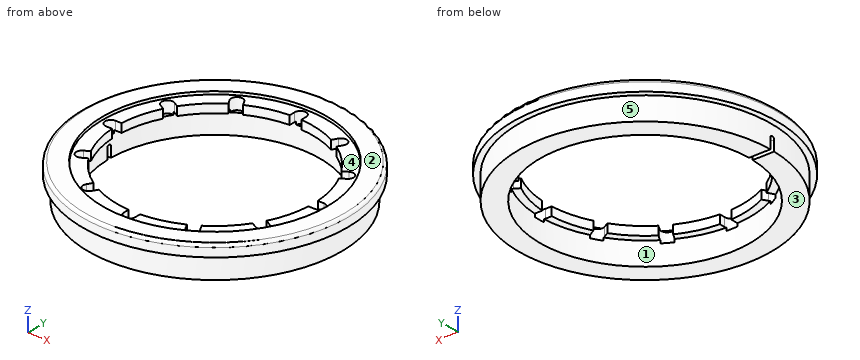
```python
from build123d import *

# Parameters (mm, degrees)
ESQUISSE1_R                  = 22
ESQUISSE1_R_2                = 18.3
BOSS_EXTRU_1_DEPTH           = 4
ESQUISSE2_R                  = 23
ESQUISSE2_R_2                = 19.5
BOSS_EXTRU_2_DEPTH           = 2
CONG_1_R                     = 0.5
ENL_V_MAT_EXTRU_1_REACH      = 25
ESQUISSE4_R                  = 19.5
ESQUISSE4_R_2                = 17
BOSS_EXTRU_3_DEPTH           = 1.5
ENL_V_MAT_EXTRU_2_DEPTH      = 2
R_P_TITION_CIRCULAIRE1_COUNT = 12


with BuildPart() as part:
    # Esquisse1 → Boss.-Extru.1 (new body)
    with BuildSketch(Plane.XY):
        Circle(ESQUISSE1_R)
        Circle(ESQUISSE1_R_2, mode=Mode.SUBTRACT)
    extrude(amount=BOSS_EXTRU_1_DEPTH)

    # Esquisse2 → Boss.-Extru.2 (add)
    with BuildSketch(Plane.XY.offset(4)):
        Circle(ESQUISSE2_R)
        Circle(ESQUISSE2_R_2, mode=Mode.SUBTRACT)
    extrude(amount=BOSS_EXTRU_2_DEPTH)

    # Congé1
    cong_1_edges = [part.edges().sort_by_distance(p)[0] for p in [
        (-23, 0, 6),
    ]]
    fillet(cong_1_edges, radius=CONG_1_R)

    # Esquisse3 → Enlèv. mat.-Extru.1 (cut, up to next)
    with BuildSketch(Plane(origin=(0, 0, 0), x_dir=(0, 0, -1), z_dir=(1, 0, 0)), mode=Mode.PRIVATE) as enl_v_mat_extru_1_sk1:
        with BuildLine():
            Line((0, -0.4), (-1.8, -0.4))
            ThreePointArc((-1.8, -0.4), (-2.2, 0), (-1.8, 0.4))
            Line((-1.8, 0.4), (0, 0.4))
            ThreePointArc((0, 0.4), (0.4, 0), (0, -0.4))
        make_face()
    enl_v_mat_extru_1_tool1 = extrude(enl_v_mat_extru_1_sk1.sketch, amount=-ENL_V_MAT_EXTRU_1_REACH, mode=Mode.PRIVATE) & part.part
    add(enl_v_mat_extru_1_tool1.solids().sort_by_distance((0, 0, 0.9))[0], mode=Mode.SUBTRACT)

    # Esquisse4 → Boss.-Extru.3 (add)
    with BuildSketch(Plane.XY.offset(4)):
        Circle(ESQUISSE4_R)
        Circle(ESQUISSE4_R_2, mode=Mode.SUBTRACT)
    extrude(amount=BOSS_EXTRU_3_DEPTH)

    # Esquisse5 → Enlèv. mat.-Extru.2 (cut)
    with BuildSketch(Plane.XY.offset(5.5)):
        with BuildLine():
            Line((-1, 15.094284231), (-1, 18))
            ThreePointArc((-1, 18), (0, 19), (1, 18))
            Line((1, 18), (1, 15.094284231))
            ThreePointArc((1, 15.094284231), (0, 14.094284231), (-1, 15.094284231))
        make_face()
    enl_v_mat_extru_2 = extrude(amount=-ENL_V_MAT_EXTRU_2_DEPTH, mode=Mode.SUBTRACT)

    # Répétition circulaire1: Enlèv. mat.-Extru.2 ×12 about axis
    r_p_tition_circulaire1_axis = Axis((0, 0, 0), (0, 0, 1))
    for i in range(1, R_P_TITION_CIRCULAIRE1_COUNT):
        add(enl_v_mat_extru_2.rotate(r_p_tition_circulaire1_axis, i * 360 / R_P_TITION_CIRCULAIRE1_COUNT), mode=Mode.SUBTRACT)


solid = part.part
```
Model file for the job. Use its own axes, mm. Face numbers are marked on the shaded views. A direction names the side the tool comes from. Coordinates: 2 decimals unless noted, no trailing zeros. Loops run counter-clockwise (first coordinate to the right, second up) from the corner with the lowest first, then second, coordinate; pieces in that order, holes last. Notation, with made-up numbers: (41.25, 8) - (66.25, 8) arc R23 ccw to (66.25, 34) - close; hole circle Ø6 at (33, 44.25). An arc over 180 degrees is marked (long way). Answer as a JSON object with one key per item and string values. Group by question number.
(1) Probe line 1 along Y through (x, z) = (0, 1.5); line 2 along X through (y, z) = (0, 2); line 3 along Y through (x, z) = (0, 5.8). List the from-to ranges inside material, lowest first.
(2) Tool access for the marked faces 1 and 2: list every direction of +Z, -Z, +X, -X, +Y, -Y with a clear straight run to the whole face (end or side of a thin tool).
(3) Cut at A-A (x = 0). Give the cut face in (y, z), then the cut area to 3 significant figures.
(4) Flat gauge pins, fed straight in: pin 1 (1.1 mm diameter, centred on x = 17.5, z = 4.5, fed in from -Y); pin 2 (2 mm diameter, centred on x = -20, z = 1, fed in from +Y); pin 3 (0.8 mm diameter, centred on x = 18.5, y = 0, fed in from +Z). Where does each tip first touch, or does it go through?
(5) Two-plate mould, pull along X, no slides. Class the marked faces 3, 4 and 5: released by +X, released by -X, zero draft, split by the parting line, or undercut.
Geometry says:
{
 "1": {"line 1": "y = -22 to -18.3, 18.3 to 22", "line 2": "x = 18.3 to 22", "line 3": "y = -22.9 to -19.5, 19.5 to 22.9"},
 "2": {"face 1": "-Z", "face 2": "+Z, +X, -X, +Y, -Y"},
 "3": {"outline": "(-23, 4) - (-22, 4) - (-22, 0) - (-18.3, 0) - (-18.3, 3.5) - (-19, 3.5) - (-19, 5.5) - (-19.5, 5.5) - (-19.5, 6) - (-22.5, 6) arc R0.5 ccw to (-23, 5.5) - close; (18.3, 0) - (22, 0) - (22, 4) - (23, 4) - (23, 5.5) arc R0.5 ccw to (22.5, 6) - (19.5, 6) - (19.5, 5.5) - (19, 5.5) - (19, 3.5) - (18.3, 3.5) - close", "area": "44.3 mm^2"},
 "4": {"pin 1": "stops at y = -15.55", "pin 2": "stops at y = 11.09", "pin 3": "stops at z = 3.5"},
 "5": {"face 3": "zero draft", "face 4": "undercut", "face 5": "split by the parting line"}
}
